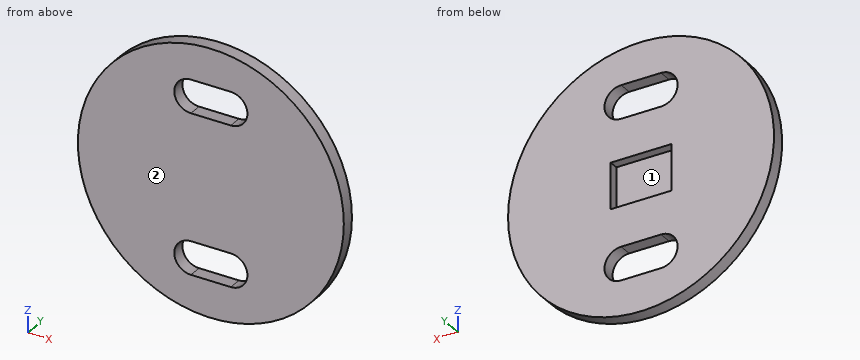
from build123d import *

# Parameters (mm, degrees)
SKETCH1_R           = 100
BOSS_EXTRUDE1_DEPTH = 10
CUT_EXTRUDE1_DEPTH  = 11
CUT_EXTRUDE2_DEPTH  = 7


with BuildPart() as part:
    # Sketch1 → Boss-Extrude1 (new body)
    with BuildSketch(Plane(origin=(0, 0, 0), x_dir=(1, 0, 0), z_dir=(0, 1, 0))):
        Circle(SKETCH1_R)
    extrude(amount=BOSS_EXTRUDE1_DEPTH)

    # Sketch2 → Cut-Extrude1 (cut, through all)
    with BuildSketch(Plane(origin=(0, 10, 0), x_dir=(1, 0, 0), z_dir=(0, 1, 0))):
        with BuildLine():
            Line((-15, -47.5), (15, -47.5))
            ThreePointArc((15, -47.5), (27.5, -60), (15, -72.5))
            Line((15, -72.5), (-15, -72.5))
            ThreePointArc((-15, -72.5), (-27.5, -60), (-15, -47.5))
        make_face()
    cut_extrude1 = extrude(amount=-CUT_EXTRUDE1_DEPTH, mode=Mode.SUBTRACT)

    # Mirror1: Cut-Extrude1 across plane
    add(cut_extrude1.mirror(Plane.XY), mode=Mode.SUBTRACT)

    # Sketch3 → Cut-Extrude2 (cut)
    with BuildSketch(Plane(origin=(0, 10, 0), x_dir=(1, 0, 0), z_dir=(0, 1, 0))):
        Polygon((-22.8, 17.3), (-22.8, -17.3), (0, 0), align=None)
        Polygon((-22.8, 17.3), (0, 0), (22.8, 17.3), align=None)
        Polygon((22.8, 17.3), (0, 0), (22.8, -17.3), align=None)
        Polygon((0, 0), (-22.8, -17.3), (22.8, -17.3), align=None)
    extrude(amount=-CUT_EXTRUDE2_DEPTH, mode=Mode.SUBTRACT)


solid = part.part
Could you check a few things on this model? Use its own coordinates, in mm. Face numbers are marked on the shaded views. Coordinates: 2 decimals unless noted, no trailing zeros. Order: outer loops, then holes, each group sorted by start corner. A loop starts at its lowest first (then second) coordinate and runs counter-clockwise, first axis right, second up.
Q1. Suppose I cut it at D-D on z = 0. Please give me the cut outline in (x, y).
Q2. Suppose I cut it at C-C on y = 8. Please give me the cut outline in (x, z), and give its area (3 significant figures).
Q3. Please list where these lines run through material, in increasing order: L1, parallel to Z at x = 9.5, y = 2.25; L2, parallel to Z at x = -11.5, y = 8.5; L3, parallel to X at y = 9.75, z = -8.5.
Q4. Thinking about a two-plate mould opening in Z: for the marked faces 1 and 2, which applies, released by +Z, released by -Z, zero draft, split by the parting line, or undercut?
Q5. Suppose I cut it at B-B on z = -60. Please give me the cut outline in (x, y), and give its area (3 significant figures).
Q6. Suppose I cut it at A-A on x = 0. Please give me the cut outline in (y, z), and give its area (3 significant figures).
Q7. Will these pins go through, and if not, where does the flat tip stop? pin 1 (6 mm diameter, centred on x = 5, y = 4, fed in from -Z); pin 2 (3 mm diameter, centred on x = -36, z = -74, fed in from -Y); pin 3 (2 mm diameter, centred on y = 7, z = -5, fed in from +X); pin 4 (6 mm diameter, centred on y = 2, z = 14.5, fed in from -X).
Answer:
1. outline: (-100, 0) - (100, 0) - (100, 10) - (22.8, 10) - (22.8, 3) - (-22.8, 3) - (-22.8, 10) - (-100, 10) - close
2. outline: circle Ø200 at (0, 0); hole (-22.8, -17.3) - (22.8, -17.3) - (22.8, 17.3) - (-22.8, 17.3) - close; hole (-15, -72.5) - (15, -72.5) arc R12.5 ccw to (15, -47.5) - (-15, -47.5) arc R12.5 ccw to start; hole (-15, 47.5) - (15, 47.5) arc R12.5 ccw to (15, 72.5) - (-15, 72.5) arc R12.5 ccw to start
2. area: 27,400 mm2
3. L1: z = -99.55 to -72.5, -47.5 to 47.5, 72.5 to 99.55
3. L2: z = -99.34 to -72.5, -47.5 to -17.3, 17.3 to 47.5, 72.5 to 99.34
3. L3: x = -99.64 to -22.8, 22.8 to 99.64
4. face 1: undercut
4. face 2: zero draft
5. outline: (-80, 0) - (-27.5, 0) - (-27.5, 10) - (-80, 10) - close; (27.5, 0) - (80, 0) - (80, 10) - (27.5, 10) - close
5. area: 1,050 mm2
6. outline: (0, -100) - (10, -100) - (10, -72.5) - (0, -72.5) - close; (0, -47.5) - (10, -47.5) - (10, -17.3) - (3, -17.3) - (3, 17.3) - (10, 17.3) - (10, 47.5) - (0, 47.5) - close; (0, 72.5) - (10, 72.5) - (10, 100) - (0, 100) - close
6. area: 1,260 mm2
7. pin 1: stops at z = -99.98
7. pin 2: stops at y = 0
7. pin 3: stops at x = 99.92
7. pin 4: stops at x = -99.34
